```python
from build123d import *

# Parameters (mm, degrees)
SKETCH1_R                                       = 5
SKETCH1_R_2                                     = 1.6
SKETCH1_R_3                                     = 1.25
SKETCH1_R_4                                     = 1.55
BOSS_EXTRUDE1_DEPTH                             = 3.18
CHAMFER1_SIZE                                   = 2.5
CHAMFER1_SIZE2                                  = 4.998920521
CSK_FOR_M2_FLAT_HEAD_MACHINE_SCREW1_D           = 2.4
CSK_FOR_M2_FLAT_HEAD_MACHINE_SCREW1_DEPTH       = 3.508967257
CSK_FOR_M2_FLAT_HEAD_MACHINE_SCREW1_CSINK_D     = 4.4
CSK_FOR_M2_FLAT_HEAD_MACHINE_SCREW1_CSINK_ANGLE = 90
CSK_FOR_M2_FLAT_HEAD_MACHINE_SCREW1_TIP         = 0.721032743
SKETCH3_R                                       = 5
CUT_EXTRUDE4_DEPTH                              = 67.382158748
FILLET2_R                                       = 3
CHAMFER2_SIZE                                   = 1.8
FILLET4_R                                       = 0.5


with BuildPart() as part:
    # Sketch1 → Boss-Extrude1 (new body)
    with BuildSketch(Plane(origin=(0, 0, 0), x_dir=(0, 0, -1), z_dir=(1, 0, 0))):
        Polygon((0, 0), (0, 30.2), (2, 32.2), (2, 61.31), (22, 61.31), (22, 41.31), (23.8, 41.31), (23.8, 24.71), (14.6, 24.71), (14.6, 13.26), (12.25, 13.26), (12.25, 11.86), (25.25, 11.86), (25.25, 6.86), (12, 6.86), (12, 0), align=None)
        with Locations(Location((7, 25.2, 0), (0, 0, 180))):
            Circle(SKETCH1_R, mode=Mode.SUBTRACT)
        with Locations(Location((7, 56.81, 0), (0, 0, 180))):
            Circle(SKETCH1_R_2, mode=Mode.SUBTRACT)
        with Locations(Location((17, 54.81, 0), (0, 0, 180))):
            Circle(SKETCH1_R_2, mode=Mode.SUBTRACT)
        with Locations(Location((22, 9.36, 0), (0, 0, 180))):
            Circle(SKETCH1_R_3, mode=Mode.SUBTRACT)
        with Locations(Location((15.5, 9.36, 0), (0, 0, 180))):
            Circle(SKETCH1_R_3, mode=Mode.SUBTRACT)
        with Locations(Location((2.55, 2.55, 0), (0, 0, 180))):
            Circle(SKETCH1_R_4, mode=Mode.SUBTRACT)
        with Locations(Location((2.55, 8.55, 0), (0, 0, 180))):
            Circle(SKETCH1_R_4, mode=Mode.SUBTRACT)
    extrude(amount=BOSS_EXTRUDE1_DEPTH)

    # Chamfer1
    chamfer1_edges = [part.edges().sort_by_distance(p)[0] for p in [
        (1.59, 0, -12),
    ]]
    chamfer1_side = [part.faces().sort_by_distance(p)[0] for p in [
        (1.59, 0, -6),
    ]]
    chamfer(chamfer1_edges, length=CHAMFER1_SIZE, length2=CHAMFER1_SIZE2, reference=chamfer1_side[0])

    # CSK for M2 Flat Head Machine Screw1
    with Locations(Plane.ZY):
        with Locations((-6.974936087, 46.414674329), (-17.432559713, 42.244769284), (-8.592504199, 35.273154083)):
            CounterSinkHole(CSK_FOR_M2_FLAT_HEAD_MACHINE_SCREW1_D / 2, CSK_FOR_M2_FLAT_HEAD_MACHINE_SCREW1_CSINK_D / 2, depth=CSK_FOR_M2_FLAT_HEAD_MACHINE_SCREW1_DEPTH, counter_sink_angle=CSK_FOR_M2_FLAT_HEAD_MACHINE_SCREW1_CSINK_ANGLE)
            with Locations((0, 0, -(CSK_FOR_M2_FLAT_HEAD_MACHINE_SCREW1_DEPTH + CSK_FOR_M2_FLAT_HEAD_MACHINE_SCREW1_TIP / 2))):  # 118° drill point
                Cone(0, CSK_FOR_M2_FLAT_HEAD_MACHINE_SCREW1_D / 2, CSK_FOR_M2_FLAT_HEAD_MACHINE_SCREW1_TIP, mode=Mode.SUBTRACT)

    # Sketch3 → Cut-Extrude4 (cut, through all)
    with BuildSketch(Plane.ZY):
        with Locations((-11, 41.310865899)):
            Circle(SKETCH3_R)
    extrude(amount=-CUT_EXTRUDE4_DEPTH, mode=Mode.SUBTRACT)

    # Fillet2
    fillet2_edges = [part.edges().sort_by_distance(p)[0] for p in [
        (1.59, 30.2, 0),
        (1.59, 32.2, -2),
    ]]
    fillet(fillet2_edges, radius=FILLET2_R)

    # Chamfer2
    chamfer2_edges = [part.edges().sort_by_distance(p)[0] for p in [
        (1.59, 61.31, -22),
        (1.59, 61.31, -2),
        (1.59, 41.31, -23.8),
    ]]
    chamfer(chamfer2_edges, length=CHAMFER2_SIZE - 0.0001)  # a hair under: the kernel refuses the full size

    # Fillet4
    fillet4_edges = [part.edges().sort_by_distance(p)[0] for p in [
        (1.59, 39.5101, -23.8),
        (1.59, 59.5101, -22),
        (1.59, 59.5101, -2),
        (1.59, 0, 0),
        (1.59, 4.998920521, -12),
    ]]
    fillet(fillet4_edges, radius=FILLET4_R)


solid = part.part
```
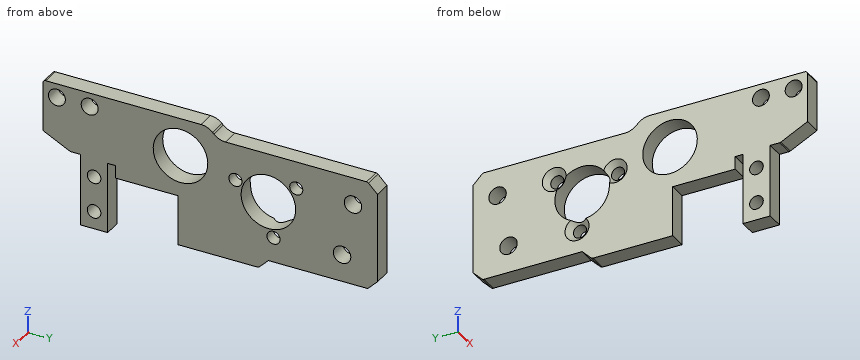
The model under review builds one solid part; all positions refer to its coordinate system, in mm. Round coordinates to 2 decimals unless told otherwise and drop trailing zeros. Loops run counter-clockwise (first coordinate to the right, second up) from the corner with the lowest first, then second, coordinate; pieces in that order, holes last. Notation, with made-up numbers: M -28.75,61 L -22.75,61 A11 ccw -22.75,71 Z; hole C 77,-11 d9. An arc over 180 degrees is marked long. Put each result on its own line as item: value.
Q1. Consider section C-C, the plane y = 38. Give the boundary of the cut face in (x, z), then the cut area to 3 significant figures.
Result set:
outline: M 0,-23.8 L 3.18,-23.8 L 3.18,-14.75 L 0,-14.75 Z; M 0,-7.25 L 3.18,-7.25 L 3.18,-2 L 0,-2 Z
area: 45.5 mm²
Q2. Consider section B-B, the plane z = -2.75. Give the boundary of the cut face in (x, y).
Result set:
outline: M 0,0 L 3.18,0 L 3.18,1.01 L 0,1.01 Z; M 0,4.09 L 3.18,4.09 L 3.18,7.01 L 0,7.01 Z; M 0,10.09 L 3.18,10.09 L 3.18,22.57 L 0,22.57 Z; M 0,27.83 L 3.18,27.83 L 3.18,60.26 L 0,60.26 Z
Q3. To check wall thickness, follow L1, parallel to Z at x = 1.4, y = 56.81; L2, parallel to Y at x = 2, z = -1.75; L3, parallel to Y at x = 0.25, z = -7. State the ranges of each line that lie inside material, in increasing order.
Result set:
L1: z = -22 to -8.6, -5.4 to -2
L2: y = 0 to 1.22, 3.88 to 7.22, 9.88 to 32.24
L3: y = 0 to 20.2, 30.2 to 34.15, 36.4 to 38.31, 44.31 to 44.46, 48.36 to 55.21, 58.41 to 61.31
Q4. Consider section A-A, the plane y = 9.36. Give the boundary of the cut face in (x, z), then the cut area to 3 significant figures.
Result set:
outline: M 0,-25.25 L 3.18,-25.25 L 3.18,-23.25 L 0,-23.25 Z; M 0,-20.75 L 3.18,-20.75 L 3.18,-16.75 L 0,-16.75 Z; M 0,-14.25 L 3.18,-14.25 L 3.18,-3.87 L 0,-3.87 Z; M 0,-1.23 L 3.18,-1.23 L 3.18,0 L 0,0 Z
area: 56.0 mm²
Q5. Consider section D-D, the plane x = 2.7. Count the separate pieces of the cut face and the enclosed holes in it, then the cut area to 3 significant figures.
Result set:
separate pieces: 1
enclosed holes: 11
area: 945 mm²
Q6. For pin 1 (1.9 mm diameter, centred on y = 35.27, z = -8.59, fed in from -X); pin 2 (1 mm diameter, centred on x = 1, y = 17, fed in from -Z); pin 3 (0.7 mm diameter, centred on x = 2, z = -13.5, fed in from -Y), all flat-tipped, find the tip position at first contact; note any pin that passes through.
Result set:
pin 1: passes through
pin 2: stops at z = -14.6
pin 3: stops at y = 6.86
